```python
from build123d import *

# Parameters (mm, degrees)
BOSS_EXTRUDE1_DEPTH = 6.35
SKETCH2_R           = 2.325
CUT_EXTRUDE1_DEPTH  = 170.824387236
SKETCH5_R           = 1.025
CUT_EXTRUDE2_DEPTH  = 170.824387236


with BuildPart() as part:
    # Sketch1 → Boss-Extrude1 (new body)
    with BuildSketch(Plane(origin=(0, 0, 0), x_dir=(1, 0, 0), z_dir=(0, 1, 0))):
        with BuildLine():
            Line((10, 0), (110, 0))
            ThreePointArc((110, 0), (117.071067812, 2.928932188), (120, 10))
            Line((120, 10), (120, 110))
            ThreePointArc((120, 110), (117.071067812, 117.071067812), (110, 120))
            Line((110, 120), (10, 120))
            ThreePointArc((10, 120), (2.928932188, 117.071067812), (0, 110))
            Line((0, 110), (0, 10))
            ThreePointArc((0, 10), (2.928932188, 2.928932188), (10, 0))
        make_face()
    extrude(amount=BOSS_EXTRUDE1_DEPTH)

    # Sketch2 → Cut-Extrude1 (cut, through all)
    with BuildSketch(Plane(origin=(0, 6.35, 0), x_dir=(1, 0, 0), z_dir=(0, 1, 0))):
        with Locations(Location((62.192235265, 7.325, 0), (0, 0, 270))):
            Circle(SKETCH2_R)
        with Locations(Location((99.974668934, 7.325, 0), (0, 0, 270))):
            Circle(SKETCH2_R)
        with Locations(Location((109.393095317, 84.031927265, 0), (0, 0, 270))):
            Circle(SKETCH2_R)
        Polygon((60.471691743, 18.506055104), (77.505195351, 8.02465468), (116.066267511, 70.690914453), (99.032763904, 81.172314877), align=None)
    extrude(amount=-CUT_EXTRUDE1_DEPTH, mode=Mode.SUBTRACT)

    # Sketch5 → Cut-Extrude2 (cut, through all)
    with BuildSketch(Plane(origin=(0, 6.35, 0), x_dir=(1, 0, 0), z_dir=(0, 1, 0))):
        with Locations(Location((69.859976402, 47.120111286, 0), (0, 0, 270))):
            Circle(SKETCH5_R)
        with Locations(Location((59.639874237, 53.408951541, 0), (0, 0, 270))):
            Circle(SKETCH5_R)
        with Locations(Location((77.72102672, 59.895238992, 0), (0, 0, 270))):
            Circle(SKETCH5_R)
        with Locations(Location((67.500924556, 66.184079246, 0), (0, 0, 270))):
            Circle(SKETCH5_R)
        with Locations(Location((13.977019656, 80.332987484, 0), (0, 0, 270))):
            Circle(SKETCH5_R)
        with Locations(Location((24.197121821, 74.04414723, 0), (0, 0, 270))):
            Circle(SKETCH5_R)
        with Locations(Location((33.106312181, 88.522625296, 0), (0, 0, 270))):
            Circle(SKETCH5_R)
        with Locations(Location((22.886210017, 94.811465551, 0), (0, 0, 270))):
            Circle(SKETCH5_R)
    extrude(amount=-CUT_EXTRUDE2_DEPTH, mode=Mode.SUBTRACT)


solid = part.part
```
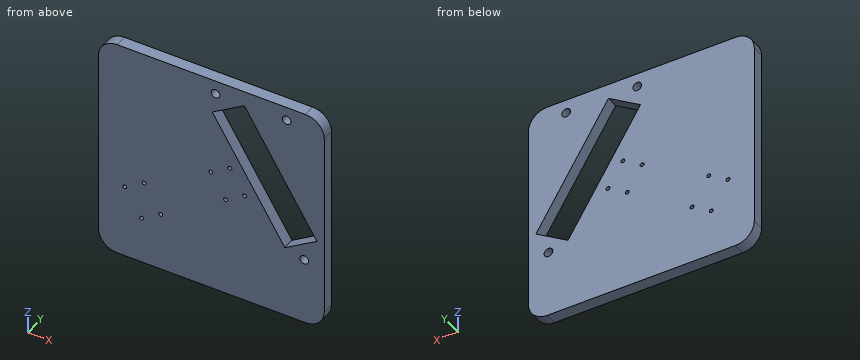
Work out the finished part from the listing and answer in its coordinate system (mm). Round coordinates to 2 decimals unless told otherwise and drop trailing zeros. Write each loop counter-clockwise with the first axis right and the second up, starting at its lowest first coordinate (ties: lowest second). Pieces come first, ordered by that corner, then holes.
1) Consider probe 1 along Z at (x, y) = (102, 3.75); probe 2 along Z at (x, y) = (64, 6); probe 3 along X at (y, z) = (5, -74.5). Determine where each line is inside the solid, lowest interval first.
2) A cutting plane is placed at B-B on x = 81. Determine the outline of the cut face in (y, z), and give its area (3 significant figures).
3) A cutting plane is placed at A-A on y = 2.75. Give the number of separate pieces and of enclosed holes in the cut face, and give its area (3 significant figures).
4) Flat-ended cylindrical pins translate along their axes: P1, Ø3.5, axis at x = 22.89, z = -94.81, coming from the -Y side; P2, Ø1.2, axis at x = 67.5, z = -66.18, coming from the +Y side. Find the tip coordinate at first contact, or state that the pin passes through.
Entries:
1. probe 1: z = -120 to -79.35, -47.83 to -8.47, -6.18 to 0
1. probe 2: z = -120 to -24.24, -16.33 to -8.79, -5.86 to 0
1. probe 3: x = 0 to 23.28, 25.12 to 94.93, 109.88 to 120
2. outline: (0, -120) - (6.35, -120) - (6.35, -51.87) - (0, -51.87) - close; (0, -13.7) - (6.35, -13.7) - (6.35, 0) - (0, 0) - close
2. area: 520 mm2
3. separate pieces: 1
3. enclosed holes: 12
3. area: 12,800 mm2
4. P1: stops at y = 0
4. P2: passes through
